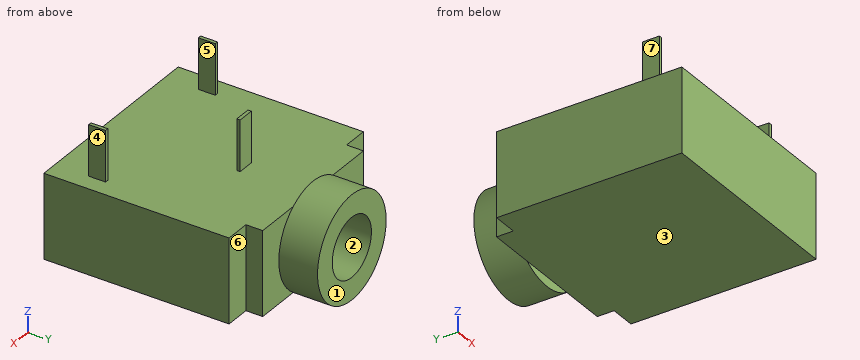
from build123d import *

# Parameters (mm, degrees)
F1_DEPTH = 5
F2_R     = 3.065
F3_DEPTH = 2.3
F4_R     = 1.75
F5_DEPTH = 8
F6_W     = 0.2
F6_H     = 1
F6_W_2   = 1
F6_H_2   = 0.2
F7_DEPTH = 3


with BuildPart() as f1:
    # F0 (on Top) → F1 (new body)
    with BuildSketch(Plane.XY):
        Polygon((6, -5.5), (6, 5.5), (4.5, 5.5), (4.5, 6.5), (-4.5, 6.5), (-4.5, 5.5), (-6, 5.5), (-6, -5.5), align=None)
    extrude(amount=F1_DEPTH)

    # F2 (on face) → F3 (join)
    with BuildSketch(Plane(origin=(0, 6.5, 0), x_dir=(-1, 0, 0), z_dir=(0, 1, 0))):
        with Locations((0, 2.5)):
            Circle(F2_R)
    extrude(amount=F3_DEPTH)

    # F4 (on face) → F5 (cut)
    with BuildSketch(Plane(origin=(0, 8.8, 0), x_dir=(-1, 0, 0), z_dir=(0, 1, 0))):
        with Locations((0, 2.5)):
            Circle(F4_R)
    extrude(amount=-F5_DEPTH, mode=Mode.SUBTRACT)

    # F6 (on face) → F7 (join)
    with BuildSketch(Plane.XY.offset(5)):
        with Locations((4.9, -3)):
            Rectangle(F6_W, F6_H)
        with Locations((-4.9, -3)):
            Rectangle(F6_W, F6_H)
        with Locations((0, 2.4)):
            Rectangle(F6_W_2, F6_H_2)
    extrude(amount=F7_DEPTH)


solid = f1.part
The model under review builds one solid part; all positions refer to its coordinate system, in mm. Face numbers are marked on the shaded views. A direction names the side the tool comes from. Round coordinates to 2 decimals unless told otherwise and drop trailing zeros. Loops run counter-clockwise (first coordinate to the right, second up) from the corner with the lowest first, then second, coordinate; pieces in that order, holes last. Notation, with made-up numbers: M 56.5,55.25 L 100.5,55.25 A23 cw 100.5,74.25 Z; hole C 42,-28 d6. An arc over 180 degrees is marked long. Answer as a JSON object with one key per item and string values.
Item 1: The part is to be moulded in two halves that separate along Z. For the marked faces 1, 2 and 3, say which applies: +Z half, -Z half, draft (parallel to the pull), parting line (faces both ways), or undercut.
Check sheet entries:
{"face 1": "draft", "face 2": "undercut", "face 3": "-Z half"}
Item 2: We need section A-A, the plane y = 3.5. State the section outline as (x, z) points.
Check sheet entries:
{"outline": "M -6,0 L 6,0 L 6,5 L -6,5 Z; hole C 0,2.5 d3.5"}
Item 3: We need section C-C, the plane x = 0. State the section outline as (y, z) points (3 decimals).
Check sheet entries:
{"outline": "M -5.5,0 L 6.5,0 L 6.5,-0.565 L 8.8,-0.565 L 8.8,0.75 L 0.8,0.75 L 0.8,4.25 L 8.8,4.25 L 8.8,5.565 L 6.5,5.565 L 6.5,5 L 2.5,5 L 2.5,8 L 2.3,8 L 2.3,5 L -5.5,5 Z"}
Item 4: Tool access review of the marked faces 4, 5, 6 and 7: name each direction out of +Z, -Z, +X, -X, +Y, -Y from which nothing blocks a thin tool from reaching the whole face with its end or side.
Check sheet entries:
{"face 4": "+Z, +X, +Y, -Y", "face 5": "+Z, +Y, -Y", "face 6": "+Z, -Z, +X, +Y", "face 7": "+Z, -X, +Y, -Y"}
Item 5: Clearance check with flat-ended pins moving along their axes: P1, Ø5, axis at x = 4.5, y = -2.5, coming from the -Z side; P2, Ø5, axis at x = 4, y = 0, coming from the +Z side; P3, Ø1.2, axis at x = -5, z = 3.5, coming from the +Y side. State where each tip first meets the part, or that it passes through.
Check sheet entries:
{"P1": "z = 0", "P2": "z = 5", "P3": "y = 6.5"}
Item 6: We need section D-D, the plane z = 6.75. State the section outline as (x, y) points.
Check sheet entries:
{"outline": "M -5,-3.5 L -4.8,-3.5 L -4.8,-2.5 L -5,-2.5 Z; M -0.5,2.3 L 0.5,2.3 L 0.5,2.5 L -0.5,2.5 Z; M 4.8,-3.5 L 5,-3.5 L 5,-2.5 L 4.8,-2.5 Z"}
Item 7: For line 1 along Z through (x, y) = (0, 6.75) (3 decimals); line 2 along Z through (x, y) = (0, 6); line 3 along Z through (x, y) = (4.75, 3.25), list the stretches that pass through material, from the lowest coordinate up.
Check sheet entries:
{"line 1": "-0.565 to 0.75, 4.25 to 5.565", "line 2": "0 to 0.75, 4.25 to 5", "line 3": "0 to 5"}
Item 8: We need section B-B, the plane z = 2.5. State the section outline as (x, y) points (3 decimals), and give its area (3 significant figures).
Check sheet entries:
{"outline": "M -6,-5.5 L 6,-5.5 L 6,5.5 L 4.5,5.5 L 4.5,6.5 L 3.065,6.5 L 3.065,8.8 L 1.75,8.8 L 1.75,0.8 L -1.75,0.8 L -1.75,8.8 L -3.065,8.8 L -3.065,6.5 L -4.5,6.5 L -4.5,5.5 L -6,5.5 Z", "area": "127 mm2"}
